Check sheet for the modelled part. Datum: model origin and axes. Units: mm. Face numbers are marked on the shaded views. A direction names the side the tool comes from. Round coordinates to 2 decimals unless told otherwise and drop trailing zeros. Loops run counter-clockwise (first coordinate to the right, second up) from the corner with the lowest first, then second, coordinate; pieces in that order, holes last. Notation, with made-up numbers: (-39, -14) -> (-20, -14) arc R29 ccw to (-20, 11) -> close; hole circle Ø11 at (-9.75, 41.5). An arc over 180 degrees is marked (long way). Return JSON: item names as keys, results as strings.
from build123d import *

# Parameters (mm, degrees)
CYLINDER002_R                        = 1.75
CYLINDER002_DEPTH                    = 19
CYLINDER003_R                        = 2.5
CYLINDER003_DEPTH                    = 4
CYLINDER004_R                        = 2.5
CYLINDER004_DEPTH                    = 4
BOX003_W                             = 71
BOX003_H                             = 2
BOX003_DEPTH                         = 8
BOX004_W                             = 1.5
BOX004_H                             = 9
BOX004_DEPTH                         = 3
BOX005_W                             = 1.5
BOX005_H                             = 9
BOX005_DEPTH                         = 3
BOX001_W                             = 75
BOX001_H                             = 1
BOX001_DEPTH                         = 10
BOX002_W                             = 71
BOX002_H                             = 2
BOX002_DEPTH                         = 8
EXTRUDE001_DEPTH                     = 2
SKETCH_W                             = 5
SKETCH_H                             = 25
EXTRUDE_DEPTH                        = 1.5
SKETCH004_R                          = 1.5
EXTRUDE003_DEPTH                     = 8
EXTRUDE008_DEPTH                     = 3
EXTRUDE008_ONTO_SKETCH007_ROLL_ANGLE = 90
EXTRUDE008_PLACEMENT_ANGLE           = 180
EXTRUDE007_DEPTH                     = 3
EXTRUDE007_ONTO_SKETCH006_ROLL_ANGLE = 90
EXTRUDE007_PLACEMENT_ANGLE           = 180
EXTRUDE006_DEPTH                     = 3
EXTRUDE006_ONTO_SKETCH006_ROLL_ANGLE = 90
EXTRUDE005_DEPTH                     = 3
EXTRUDE005_ONTO_SKETCH006_ROLL_ANGLE = 90
BOX_W                                = 75
BOX_H                                = 1
BOX_DEPTH                            = 10


with BuildPart() as cylinder002:
    # Cylinder002 → Cylinder002 (new body)
    with BuildSketch(Plane(origin=(24, 0, -8), x_dir=(1, 0, 0), z_dir=(0, 0, 1))):
        Circle(CYLINDER002_R)
    extrude(amount=CYLINDER002_DEPTH)


with BuildPart() as cylinder003:
    # Cylinder003 → Cylinder003 (new body)
    with BuildSketch(Plane(origin=(-12, -8, 0), x_dir=(1, 0, 0), z_dir=(0, 0, 1))):
        Circle(CYLINDER003_R)
    extrude(amount=CYLINDER003_DEPTH)


with BuildPart() as holesside1:
    # Cylinder004 → Cylinder004 (new body)
    with BuildSketch(Plane(origin=(-12, 8, 0), x_dir=(1, 0, 0), z_dir=(0, 0, 1))):
        Circle(CYLINDER004_R)
    extrude(amount=CYLINDER004_DEPTH)

    # Fusion005: union Cylinder002, Cylinder003
    add(cylinder002.part)
    add(cylinder003.part)


with BuildPart() as sidewall004:
    # Box003 → Box003 (new body)
    with BuildSketch(Plane(origin=(-25, 15, 1.5), x_dir=(1, 0, 0), z_dir=(0, 0, 1))):
        with Locations((35.5, 1)):
            Rectangle(BOX003_W, BOX003_H)
    extrude(amount=BOX003_DEPTH)


with BuildPart() as cube:
    # Box004 → Box004 (new body)
    with BuildSketch(Plane(origin=(48.5, 9, 1.5), x_dir=(1, 0, 0), z_dir=(0, 0, 1))):
        with Locations((0.75, 4.5)):
            Rectangle(BOX004_W, BOX004_H)
    extrude(amount=BOX004_DEPTH)


with BuildPart() as cube001:
    # Box005 → Box005 (new body)
    with BuildSketch(Plane(origin=(48.5, -18, 1.5), x_dir=(1, 0, 0), z_dir=(0, 0, 1))):
        with Locations((0.75, 4.5)):
            Rectangle(BOX005_W, BOX005_H)
    extrude(amount=BOX005_DEPTH)


with BuildPart() as sidewall002:
    # Box001 → Box001 (new body)
    with BuildSketch(Plane(origin=(-25, 17, 1.5), x_dir=(1, 0, 0), z_dir=(0, 0, 1))):
        with Locations((37.5, 0.5)):
            Rectangle(BOX001_W, BOX001_H)
    extrude(amount=BOX001_DEPTH)


with BuildPart() as sidewall003:
    # Box002 → Box002 (new body)
    with BuildSketch(Plane(origin=(-25, -17, 1.5), x_dir=(1, 0, 0), z_dir=(0, 0, 1))):
        with Locations((35.5, 1)):
            Rectangle(BOX002_W, BOX002_H)
    extrude(amount=BOX002_DEPTH)


with BuildPart() as extrude001:
    # Sketch001 → Extrude001 (new body)
    with BuildSketch(Plane.YZ):
        Polygon((-18, 0), (18, 0), (18, 10), (13, 10), (13, 8.5), (2, 8.5), (2, 10), (-2, 10), (-2, 8.5), (-13, 8.5), (-13, 10), (-18, 10), align=None)
    extrude(amount=EXTRUDE001_DEPTH)


with BuildPart() as extrude001_1:
    # Extrude001 placement: moved
    add(extrude001.part.moved(Location((-25, 0, 1.5))))


with BuildPart() as extrude_body:
    # Sketch → Extrude (new body)
    with BuildSketch(Plane.XY):
        Polygon((-25, 18), (-25, -18), (50, -18), (50, -9), (28, -9), (28, 9), (50, 9), (50, 18), align=None)
        with Locations((2.5, 0)):
            Rectangle(SKETCH_W, SKETCH_H, mode=Mode.SUBTRACT)
    extrude(amount=EXTRUDE_DEPTH)


with BuildPart() as extrude003:
    # Sketch004 → Extrude003 (new body)
    with BuildSketch(Plane.XY):
        Polygon((-3, 13), (11, 13), (11, 5), (0, 5), (0, -5), (11, -5), (11, -13), (-3, -13), align=None)
        with Locations((8, 8)):
            Circle(SKETCH004_R, mode=Mode.SUBTRACT)
        with Locations((8, -8)):
            Circle(SKETCH004_R, mode=Mode.SUBTRACT)
    extrude(amount=EXTRUDE003_DEPTH)


with BuildPart() as extrude003_1:
    # Extrude003 placement: moved
    add(extrude003.part.moved(Location((-20, 0, 0))))


with BuildPart() as extrude008:
    # Sketch007 as drawn → Extrude008 (new)
    with BuildSketch(Plane.XY):
        Polygon((0, 0), (-1.5, 0), (-1.5, 5.5), (0, 5.5), (0.5, 3), (0, 2), align=None)
    extrude(amount=EXTRUDE008_DEPTH)


with BuildPart() as extrude008_1:
    # Extrude008 onto Sketch007 roll: moved
    add(extrude008.part.rotate(Axis((0, 0, 0), (1, 0, 0)), EXTRUDE008_ONTO_SKETCH007_ROLL_ANGLE))


with BuildPart() as extrude008_2:
    # Extrude008 onto Sketch007 placement: moved
    add(extrude008_1.part)


with BuildPart() as extrude008_3:
    # Extrude008 placement: moved
    add(extrude008_2.part.moved(Location((10.5, -11, 1.5))).rotate(Axis((10.5, -11, 1.5), (0, 0, 1)), EXTRUDE008_PLACEMENT_ANGLE))


with BuildPart() as extrude007:
    # Sketch006 as drawn → Extrude007 (new)
    with BuildSketch(Plane.XY):
        Polygon((0, 0), (-1.5, 0), (-1.5, 5.5), (0, 5.5), (0.5, 3), (0, 2), align=None)
    extrude(amount=EXTRUDE007_DEPTH)


with BuildPart() as extrude007_1:
    # Extrude007 onto Sketch006 roll: moved
    add(extrude007.part.rotate(Axis((0, 0, 0), (1, 0, 0)), EXTRUDE007_ONTO_SKETCH006_ROLL_ANGLE))


with BuildPart() as extrude007_2:
    # Extrude007 onto Sketch006 placement: moved
    add(extrude007_1.part)


with BuildPart() as extrude007_3:
    # Extrude007 placement: moved
    add(extrude007_2.part.moved(Location((10.5, 8, 1.5))).rotate(Axis((10.5, 8, 1.5), (0, 0, 1)), EXTRUDE007_PLACEMENT_ANGLE))


with BuildPart() as extrude006:
    # Sketch006 as drawn → Extrude006 (new)
    with BuildSketch(Plane.XY):
        Polygon((0, 0), (-1.5, 0), (-1.5, 5.5), (0, 5.5), (0.5, 3), (0, 2), align=None)
    extrude(amount=EXTRUDE006_DEPTH)


with BuildPart() as extrude006_1:
    # Extrude006 onto Sketch006 roll: moved
    add(extrude006.part.rotate(Axis((0, 0, 0), (1, 0, 0)), EXTRUDE006_ONTO_SKETCH006_ROLL_ANGLE))


with BuildPart() as extrude006_2:
    # Extrude006 onto Sketch006 placement: moved
    add(extrude006_1.part)


with BuildPart() as extrude006_3:
    # Extrude006 placement: moved
    add(extrude006_2.part.moved(Location((-6, -8, 1.5))))


with BuildPart() as pcb_holder:
    # Sketch006 as drawn → Extrude005 (new)
    with BuildSketch(Plane.XY):
        Polygon((0, 0), (-1.5, 0), (-1.5, 5.5), (0, 5.5), (0.5, 3), (0, 2), align=None)
    extrude(amount=EXTRUDE005_DEPTH)


with BuildPart() as pcb_holder_1:
    # Extrude005 onto Sketch006 roll: moved
    add(pcb_holder.part.rotate(Axis((0, 0, 0), (1, 0, 0)), EXTRUDE005_ONTO_SKETCH006_ROLL_ANGLE))


with BuildPart() as pcb_holder_2:
    # Extrude005 onto Sketch006 placement: moved
    add(pcb_holder_1.part)


with BuildPart() as pcb_holder_3:
    # Extrude005 placement: moved
    add(pcb_holder_2.part.moved(Location((-6, 11, 1.5))))

    # Fusion007: union Extrude008, Extrude007, Extrude006
    add(extrude008_3.part)
    add(extrude007_3.part)
    add(extrude006_3.part)


with BuildPart() as obj1:
    # Box → Box (new body)
    with BuildSketch(Plane(origin=(-25, -18, 1.5), x_dir=(1, 0, 0), z_dir=(0, 0, 1))):
        with Locations((37.5, 0.5)):
            Rectangle(BOX_W, BOX_H)
    extrude(amount=BOX_DEPTH)

    # Fusion: union sidewall004, Cube, Cube001, sidewall002, sidewall003, Extrude001, Extrude body, Extrude003, pcb_holder
    add(sidewall004.part)
    add(cube.part)
    add(cube001.part)
    add(sidewall002.part)
    add(sidewall003.part)
    add(extrude001_1.part)
    add(extrude_body.part)
    add(extrude003_1.part)
    add(pcb_holder_3.part)

    # Cut001: cut HolesSide1
    add(holesside1.part, mode=Mode.SUBTRACT)


solid = obj1.part
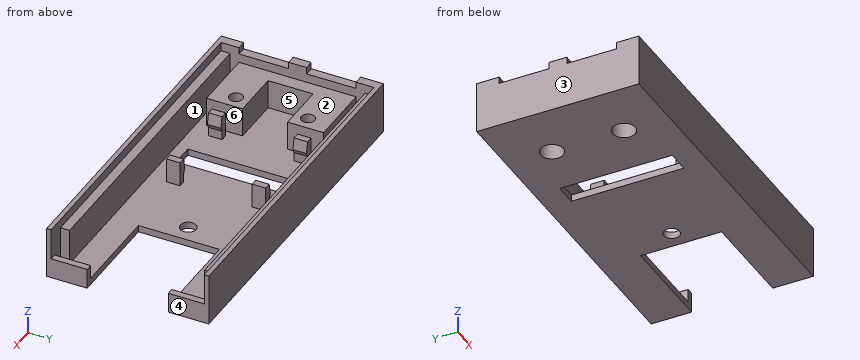
Q1. Material ranges on line 1 (Y direction, x = -12, z = 6.6); line 2 (Y direction, x = -12, z = 1.55); line 3 (Y direction, x = -12, z = 1.4), recorded low to high.
Results list:
{"line 1": "-18 to -15, -13 to -9.5, -6.5 to -5, 5 to 6.5, 9.5 to 13, 15 to 18", "line 2": "-18 to -15, -13 to -10.5, -5.5 to -5, 5 to 5.5, 10.5 to 13, 15 to 18", "line 3": "-18 to -10.5, -5.5 to 5.5, 10.5 to 18"}
Q2. Section check D-D (x = -12). Count the separate pieces of the cut face and the enclosed holes in it, then the cut area to 3 significant figures.
Results list:
{"separate pieces": "3", "enclosed holes": "0", "area": "146 mm^2"}
Q3. Section check A-A (x = 24). Record the boundary of the cut face in (y, z).
Results list:
{"outline": "(-18, 0) -> (-1.75, 0) -> (-1.75, 1.5) -> (-15, 1.5) -> (-15, 9.5) -> (-17, 9.5) -> (-17, 11.5) -> (-18, 11.5) -> close; (1.75, 0) -> (18, 0) -> (18, 11.5) -> (17, 11.5) -> (17, 9.5) -> (15, 9.5) -> (15, 1.5) -> (1.75, 1.5) -> close"}
Q4. Section check C-C (y = 0). Record the boundary of the cut face in (x, z).
Results list:
{"outline": "(-25, 0) -> (0, 0) -> (0, 1.5) -> (-20, 1.5) -> (-20, 8) -> (-23, 8) -> (-23, 11.5) -> (-25, 11.5) -> close; (5, 0) -> (22.25, 0) -> (22.25, 1.5) -> (5, 1.5) -> close; (25.75, 0) -> (28, 0) -> (28, 1.5) -> (25.75, 1.5) -> close"}
Q5. Tool access check on the marked faces 4, 5 and 6. Record the directions out of +Z, -Z, +X, -X, +Y, -Y that give a thin tool (end or side, any length) a straight path to the whole face; none if there is none.
Results list:
{"face 4": "+Z, -Z, +X, +Y, -Y", "face 5": "+Z, +X", "face 6": "+Z"}
Q6. Draft check along X on the marked faces 1, 2 and 3. Enter one of: released by +X, released by -X, zero draft, split by the parting line, or undercut.
Results list:
{"face 1": "undercut", "face 2": "zero draft", "face 3": "released by -X"}
Q7. Go/stop test with flat-tipped pins: pin 1 (8 mm diameter, centred on x = 42.5, y = -10, fed in from -Z); pin 2 (0.8 mm diameter, centred on x = 11, y = 10, fed in from +Z); pin 3 (4 mm diameter, centred on x = -12, y = -8, fed in from +Z); pin 4 (2 mm diameter, centred on y = -1, z = 4.5, fed in from +X). Record where each tip stops, or that it passes through.
Results list:
{"pin 1": "z = 0", "pin 2": "z = 7", "pin 3": "z = 8", "pin 4": "x = -20"}
Q8. Section check B-B (y = 4). Record the boundary of the cut face in (x, z).
Results list:
{"outline": "(-25, 0) -> (0, 0) -> (0, 1.5) -> (-20, 1.5) -> (-20, 8) -> (-23, 8) -> (-23, 10) -> (-25, 10) -> close; (5, 0) -> (28, 0) -> (28, 1.5) -> (5, 1.5) -> close"}
